Check sheet for the modelled part. Datum: model origin and axes. Units: mm. Face numbers are marked on the shaded views. A direction names the side the tool comes from. Round coordinates to 2 decimals unless told otherwise and drop trailing zeros. Write each loop counter-clockwise with the first axis right and the second up, starting at its lowest first coordinate (ties: lowest second). Pieces come first, ordered by that corner, then holes. Notation, with made-up numbers: (-17.5, 44) - (6.5, 44) arc R25 cw to (6.5, 83) - close; hole circle Ø10 at (72, 80). An arc over 180 degrees is marked (long way). Answer as a JSON object with one key per item and string values. Group by question number.
Item 1: Sectioned sample at C-C on z = 23.5. Count the separate pieces of the cut face and the enclosed holes in it, plus the area to 3 significant figures.
Item 2: Set-up check for the marked faces 4, 5, 6, 7 and 8: record each of +Z, -Z, +X, -X, +Y, -Y from which the full face is reachable in a straight line by a thin tool's end or side.
Item 3: Release check for a two-part mould opening along X. For the marked faces 1, 2 and 3 record: pulls with the +X half, pulls with the -X half, needs draft (parallel to the pull), parting line crosses it, or undercut.
Item 4: Sectioned sample at A-A on z = 2. Record the boundary of the cut face in (x, y).
Item 5: Gauge pin test, flat ends, axial feed: P1, Ø8, axis at x = 14.5, z = 5, coming from the -Y side; P2, Ø1.3, axis at y = -24, z = 23, coming from the -X side; P3, Ø9.5, axis at x = 20, z = 18.5, coming from the +Y side (3 decimals); P4, Ø7.5, axis at x = 26, z = 17, coming from the -Y side. Record the tip position at first contact, or that the pin passes through.
Item 6: Sectioned sample at D-D on y = -29. Record the boundary of the cut face in (x, z) (3 decimals), plus the area to 3 significant figures.
Item 7: Thickness scan on line 1 (Y direction, x = 3.5, z = 9); line 2 (Y direction, x = 27.5, z = 28.5); line 3 (X direction, y = -17, z = 17.5). Record the ranges inside material, lowest first.
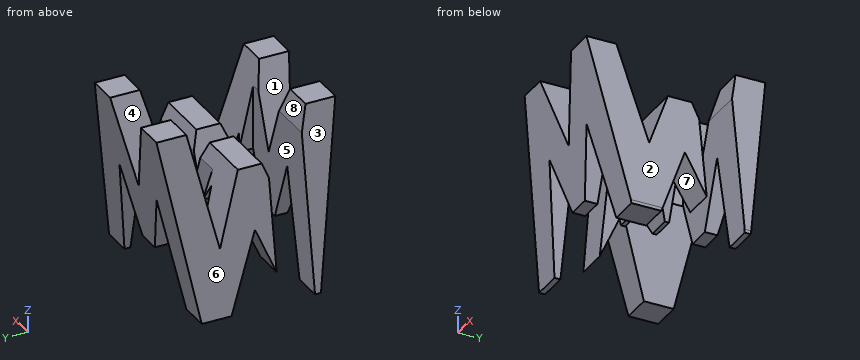
```python
from build123d import *

# Parameters (mm, degrees)
F0_W      = 37.977102
F0_H      = 38.1
F1_DEPTH  = 38.1
F6_DEPTH  = 38.1
F8_DEPTH  = 38.1
F9_W      = 25.4
F9_H      = 7.62
F10_DEPTH = 38.1


with BuildPart() as f1:
    # F0 (on Front) → F1 (new body)
    with BuildSketch(Plane.XZ):
        with Locations((18.988551, 19.05)):
            Rectangle(F0_W, F0_H)
    extrude(amount=F1_DEPTH)

    # F5 (on offset) → F6 (cut)
    with BuildSketch(Plane.YZ.offset(38.1)):
        Polygon((-31.75, 0), (-38.1, 38.1), (-38.1, 0), align=None)
        Polygon((-11.43, 13.831229), (-6.35, 38.1), (-31.75, 38.1), (-26.67, 15.875), (-21.59, 28.575), (-16.51, 28.575), align=None)
        Polygon((-19.05, 0), (-12.7, 0), (-19.05, 15.875), (-25.4, 0), align=None)
        Polygon((0, 0), (0, 38.1), (-6.35, 0), align=None)
    extrude(amount=-F6_DEPTH, mode=Mode.SUBTRACT)

    # F7 (on offset) → F8 (cut)
    with BuildSketch(Plane.XZ.offset(38.1)):
        Polygon((11.43, 22.225), (6.35, 0), (31.75, 0), (26.67, 22.225), (21.59, 8.616461), (16.51, 8.616461), align=None)
        Polygon((25.4, 38.1), (12.7, 38.1), (19.05, 21.316461), align=None)
        Polygon((0, 38.1), (0, 0), (6.35, 38.1), align=None)
        Polygon((31.75, 38.1), (38.1, 0), (38.1, 38.1), align=None)
    extrude(amount=-F8_DEPTH, mode=Mode.SUBTRACT)

    # F9 (on offset) → F10 (cut)
    with BuildSketch(Plane.XY.offset(38.1)):
        with Locations((25.4, -11.43)):
            Rectangle(F9_W, F9_H)
        with Locations((12.7, -26.67)):
            Rectangle(F9_W, F9_H)
    extrude(amount=-F10_DEPTH, mode=Mode.SUBTRACT)


solid = f1.part
```
Completed:
{
 "1": {"separate pieces": "6", "enclosed holes": "0", "area": "560 mm²"},
 "2": {"face 4": "+Z, +Y, -Y", "face 5": "+Z, -Z, -X", "face 6": "+Z, -X, +Y, -Y", "face 7": "-Z, +X, -X", "face 8": "+Z, +X, -X"},
 "3": {"face 1": "undercut", "face 2": "pulls with the +X half", "face 3": "pulls with the -X half"},
 "4": {"outline": "(0.33, -32.08) - (6.81, -32.08) - (6.81, -30.48) - (0.33, -30.48) - close; (0.33, -13.5) - (6.81, -13.5) - (6.81, -6.02) - (0.33, -6.02) - close; (31.29, -32.08) - (37.77, -32.08) - (37.77, -24.6) - (31.29, -24.6) - close; (31.29, -7.62) - (37.77, -7.62) - (37.77, -6.02) - (31.29, -6.02) - close"},
 "5": {"P1": "through", "P2": "x = 25.4", "P3": "y = -2.475", "P4": "y = -35.21"},
 "6": {"outline": "(25.4, 18.823) - (26.67, 22.225) - (31.75, 0) - (37.977, 0) - (37.977, 0.737) - (33.755, 26.069) - (25.4, 26.069) - close", "area": "192 mm²"},
 "7": {"line 1": "-33.25 to -30.48, -22.86 to -21.8, -16.3 to -4.85", "line 2": "-36.5 to -29.56, -21.62 to -16.48, -7.62 to -1.6", "line 3": "2.92 to 10.35, 13.19 to 24.91, 27.75 to 35.18"}
}
